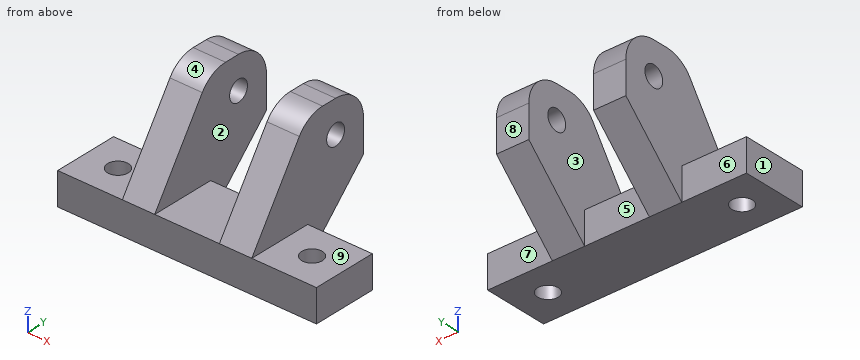
```python
from build123d import *

# Parameters (mm, degrees)
SKETCH1_W           = 40
SKETCH1_H           = 10
BOSS_EXTRUDE1_DEPTH = 5
SKETCH2_W           = 5
SKETCH2_H           = 10
BOSS_EXTRUDE2_DEPTH = 15
SKETCH4_R           = 1.6
CUT_EXTRUDE2_DEPTH  = 15
SKETCH5_W           = 5
SKETCH5_H           = 20
BOSS_EXTRUDE3_DEPTH = 10
CUT_EXTRUDE3_REACH  = 41.051
SKETCH6_R           = 1.6
CUT_EXTRUDE4_REACH  = 41.051
FILLET2_R           = 5
CUT_EXTRUDE5_REACH  = 41.051


with BuildPart() as part:
    # Sketch1 → Boss-Extrude1 (new body)
    with BuildSketch(Plane.XY):
        Rectangle(SKETCH1_W, SKETCH1_H)
    extrude(amount=BOSS_EXTRUDE1_DEPTH)

    # Sketch2 → Boss-Extrude2 (add)
    with BuildSketch(Plane.XY.offset(5)):
        with Locations((-7.5, 0)):
            Rectangle(SKETCH2_W, SKETCH2_H)
        with Locations((7.5, 0)):
            Rectangle(SKETCH2_W, SKETCH2_H)
    extrude(amount=BOSS_EXTRUDE2_DEPTH)

    # Sketch4 → Cut-Extrude2 (cut)
    with BuildSketch(Plane(origin=(0, 0, 0), x_dir=(-1, 0, 0), z_dir=(0, 0, -1))):
        with Locations((-15, 0)):
            Circle(SKETCH4_R)
        with Locations(Location((15, 0, 0), (0, 0, 180))):
            Circle(SKETCH4_R)
    extrude(amount=-CUT_EXTRUDE2_DEPTH, mode=Mode.SUBTRACT)

    # Sketch5 → Boss-Extrude3 (add)
    with BuildSketch(Plane(origin=(0, 5, 0), x_dir=(1, 0, 0), z_dir=(0, 1, 0))):
        with Locations((-7.5, -10)):
            Rectangle(SKETCH5_W, SKETCH5_H)
        with Locations((7.5, -10)):
            Rectangle(SKETCH5_W, SKETCH5_H)
    extrude(amount=BOSS_EXTRUDE3_DEPTH)

    # Cut-Extrude3: up to this face of the body (flat: up to its plane)
    cut_extrude3_end = Plane(part.part.faces().sort_by_distance((10, 5.714285714, 11.071428571))[0])
    # Sketch6 → Cut-Extrude3 (cut, up to the picked face)
    with BuildSketch(Plane.ZY.offset(10), mode=Mode.PRIVATE) as cut_extrude3_sk1:
        with Locations((15, 10)):
            Circle(SKETCH6_R)
    cut_extrude3_tool1 = split(extrude(cut_extrude3_sk1.sketch, amount=-CUT_EXTRUDE3_REACH, mode=Mode.PRIVATE), bisect_by=cut_extrude3_end, keep=Keep.BOTH, mode=Mode.PRIVATE)
    add(cut_extrude3_tool1.solids().sort_by(Axis((-10, 10, 15), (1, 0, 0)))[0], mode=Mode.SUBTRACT)

    # Cut-Extrude4: up to this face of the body (flat: up to its plane)
    cut_extrude4_end = Plane(part.part.faces().sort_by_distance((10, 5.613490273, 10.97903275))[0])
    # Sketch7 → Cut-Extrude4 (cut, up to the picked face)
    with BuildSketch(Plane.ZY.offset(10), mode=Mode.PRIVATE) as cut_extrude4_sk1:
        Polygon((20, 5), (5, -5), (20, -5), align=None)
    cut_extrude4_tool1 = split(extrude(cut_extrude4_sk1.sketch, amount=-CUT_EXTRUDE4_REACH, mode=Mode.PRIVATE), bisect_by=cut_extrude4_end, keep=Keep.BOTH, mode=Mode.PRIVATE)
    add(cut_extrude4_tool1.solids().sort_by(Axis((-10, -1.666667, 15), (1, 0, 0)))[0], mode=Mode.SUBTRACT)

    # Fillet2
    fillet2_edges = [part.edges().sort_by_distance(p)[0] for p in [
        (-7.5, 15, 20),
        (7.5, 15, 20),
        (-7.5, 5, 20),
        (7.5, 5, 20),
    ]]
    fillet(fillet2_edges, radius=FILLET2_R)

    # Cut-Extrude5: up to this face of the body (flat: up to its plane)
    cut_extrude5_end = Plane(part.part.faces().sort_by_distance((10, 7.540739084, 9.622610051))[0])
    # Sketch8 → Cut-Extrude5 (cut, up to the picked face)
    with BuildSketch(Plane.ZY.offset(10), mode=Mode.PRIVATE) as cut_extrude5_sk1:
        Polygon((0, 5), (10, 15), (0, 15), align=None)
    cut_extrude5_tool1 = split(extrude(cut_extrude5_sk1.sketch, amount=-CUT_EXTRUDE5_REACH, mode=Mode.PRIVATE), bisect_by=cut_extrude5_end, keep=Keep.BOTH, mode=Mode.PRIVATE)
    add(cut_extrude5_tool1.solids().sort_by(Axis((-10, 11.666667, 3.333333), (1, 0, 0)))[0], mode=Mode.SUBTRACT)


solid = part.part
```
Here's how the part is built. I have some questions about the finished solid (model axes, mm). Face numbers are marked on the shaded views. A direction names the side the tool comes from. Round coordinates to 2 decimals unless told otherwise and drop trailing zeros. Loops run counter-clockwise (first coordinate to the right, second up) from the corner with the lowest first, then second, coordinate; pieces in that order, holes last. Notation, with made-up numbers: (39.5, 16.25) -> (62.5, 16.25) arc R6 cw to (62.5, 24.25) -> close; hole circle Ø6 at (-28, -21). An arc over 180 degrees is marked (long way). Answer as CSV lines item,"result". Start each with the question number.
1. Imagine slicing it at A-A on y = 0. Write out the boundary of the cut face in (x, z), plus the area to 3 significant figures.
2. If we mould it in two halves opening along X, with no side actions, what happens to the marked faces 1, 2, 3 and 4? For each: pulls with the +X half, pulls with the -X half, needs draft (parallel to the pull), parting line crosses it, or undercut.
3. For the marked faces 5, 6, 7, 8 and 9, which set-ups out of +Z, -Z, +X, -X, +Y, -Y let a thin tool reach every point of the face, with its end or its side?
4. Imagine slicing it at D-D on y = 9. Write out the boundary of the cut face in (x, z), plus the area to 3 significant figures.
5. Imagine slicing it at C-C on y = 13. Write out the boundary of the cut face in (x, z), plus the area to 3 significant figures.
6. Imagine slicing it at B-B on x = 15. Write out the boundary of the cut face in (y, z).
7. I need wall thicknesses on probe 1 along X at (y, z) = (-1.25, 10.25); probe 2 along Y at (x, z) = (15, 1.4); probe 3 along Z at (x, y) = (-11.5, 3.25). Which ranges of each line are inside material? Lowest first, please. Write a range as from..to.
8. I'm going to push flat-ended pins straight in: P1, Ø2.5, axis at x = 0, z = 3.5, coming from the +Y side; P2, Ø6, axis at x = 6.5, z = 15.5, coming from the -Y side; P3, Ø5, axis at x = 13, y = 0, coming from the +Z side. Where does each tip first touch, or does it pass through?
Solution:
1,outline,"(-20, 0) -> (-16.6, 0) -> (-16.6, 5) -> (-20, 5) -> close; (-13.4, 0) -> (13.4, 0) -> (13.4, 5) -> (10, 5) -> (10, 12.5) -> (5, 12.5) -> (5, 5) -> (-5, 5) -> (-5, 12.5) -> (-10, 12.5) -> (-10, 5) -> (-13.4, 5) -> close; (16.6, 0) -> (20, 0) -> (20, 5) -> (16.6, 5) -> close"
1,area,"243 mm²"
2,face 1,"pulls with the -X half"
2,face 2,"undercut"
2,face 3,"undercut"
2,face 4,"needs draft"
3,face 5,"+Z, -Z, +Y"
3,face 6,"+Z, -Z, -X, +Y"
3,face 7,"+Z, -Z, +X, +Y"
3,face 8,"+Z, -Z, +X, -X, +Y"
3,face 9,"+Z, +X, +Y, -Y"
4,outline,"(-10, 4) -> (-5, 4) -> (-5, 13.75) -> (-10, 13.75) -> close; (-10, 16.25) -> (-5, 16.25) -> (-5, 20) -> (-10, 20) -> close; (5, 4) -> (10, 4) -> (10, 13.75) -> (5, 13.75) -> close; (5, 16.25) -> (10, 16.25) -> (10, 20) -> (5, 20) -> close"
4,area,"135 mm²"
5,outline,"(-10, 8) -> (-5, 8) -> (-5, 19) -> (-10, 19) -> close; (5, 8) -> (10, 8) -> (10, 19) -> (5, 19) -> close"
5,area,"110 mm²"
6,outline,"(-5, 0) -> (-1.6, 0) -> (-1.6, 5) -> (-5, 5) -> close; (1.6, 0) -> (5, 0) -> (5, 5) -> (1.6, 5) -> close"
7,probe 1,"-10..-5, 5..10"
7,probe 2,"-5..-1.6, 1.6..5"
7,probe 3,"0..5"
8,P1,"y = 5"
8,P2,"y = 0"
8,P3,"z = 5"
